Answer from the drawing. Dimensions are ordinates in mm from the lowest x, y and z of the part. A direction names the side the tool comes from. Give positions to 0.01 mm unless a question says otherwise; leave off trailing zeros. Write each loop counter-clockwise with the first axis right and the second up, starting at its lowest first coordinate (ties: lowest second). Pieces come first, ordered by that corner, then holes.
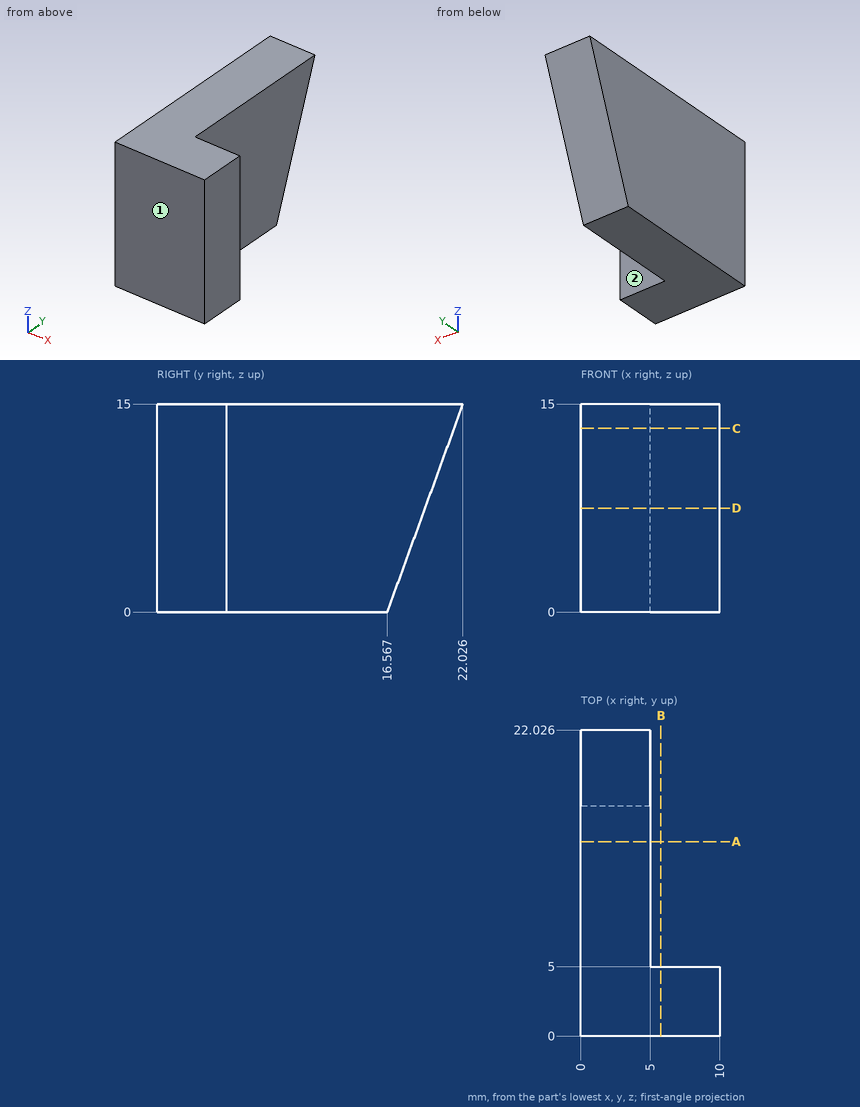
Item 1: A cutting plane is placed at C-C, the plane z = 13.25. Give the vertices of the cut face in (x, y), plus the area to 3 significant figures.
Conclusion:
outline: (0, 0) - (10, 0) - (10, 5) - (5, 5) - (5, 21.39) - (0, 21.39) - close
area: 132 mm2
Item 2: A cutting plane is placed at A-A, the plane y = 14. Give the vertices of the cut face in (x, z), plus the area to 3 significant figures.
Conclusion:
outline: (0, 0) - (5, 0) - (5, 15) - (0, 15) - close
area: 75.0 mm2
Item 3: Consider probe 1 along Y at (x, z) = (6.25, 2.5); probe 2 along Y at (x, z) = (1.25, 1). Determine where each line is inside the solid, lowest interval first.
Conclusion:
probe 1: y = 0 to 5
probe 2: y = 0 to 16.93
Item 4: A cutting plane is placed at D-D, the plane z = 7.5. Give the vertices of the cut face in (x, y).
Conclusion:
outline: (0, 0) - (10, 0) - (10, 5) - (5, 5) - (5, 19.3) - (0, 19.3) - close
Item 5: Which of the six approach directions +Z, -Z, +X, -X, +Y, -Y give full straight-line access (tool end or side, diameter ignored) to the marked faces 1 and 2?
Conclusion:
face 1: +Z, -Z, +X, -X, -Y
face 2: +Z, -Z, +X, +Y
Item 6: Each of these flat-tipped pins is pushed along its axis until it touches: P1, Ø4, axis at x = 2, z = 9, coming from the +Y side; P2, Ø5.5, axis at x = 8.5, z = 6.5, coming from the +Y side. Where does it stop, or does it pass through?
Conclusion:
P1: stops at y = 20.57
P2: stops at y = 5
